Geometry check sheet. Reference: the model listing, model coordinates, mm. Face numbers are marked on the shaded views. Round coordinates to 2 decimals unless told otherwise and drop trailing zeros. Loops run counter-clockwise (first coordinate to the right, second up) from the corner with the lowest first, then second, coordinate; pieces in that order, holes last. Notation, with made-up numbers: M 28,35.5 L 64,35.5 A6 ccw 64,39.5 Z; hole C -14.5,46.25 d1. An arc over 180 degrees is marked long. Use one line per item in the form item = value. Start each with the question number.
1. Material ranges on line 1 (Y direction, x = 0, z = 5); line 2 (Z direction, x = 0, y = -42); line 3 (X direction, y = -3, z = 4.75), recorded low to high.
2. Draft check along Y on the marked faces 1, 2 and 3. Enter one of: pulls with the +Y half, pulls with the -Y half, needs draft (parallel to the pull), parting line crosses it, or undercut.
3. Cross-section at A-A (y = 0). Record the boundary of the cut face in (x, z).
4. Cross-section at C-C (y = -16). Record the boundary of the cut face in (x, z), then the cut area to 3 significant figures.
5. Go/stop test with flat-tipped pins: pin 1 (0.9 mm diameter, centred on y = 0.5, z = 4.5, fed in from -X); pin 2 (1.5 mm diameter, centred on x = 0, z = 4, fed in from +Y); pin 3 (1.5 mm diameter, centred on y = 22, z = 6, fed in from +X). Record where each tip stops, or that it passes through.
6. Cross-section at B-B (z = 4). Record the boundary of the cut face in (x, y), then the cut area to 3 significant figures.
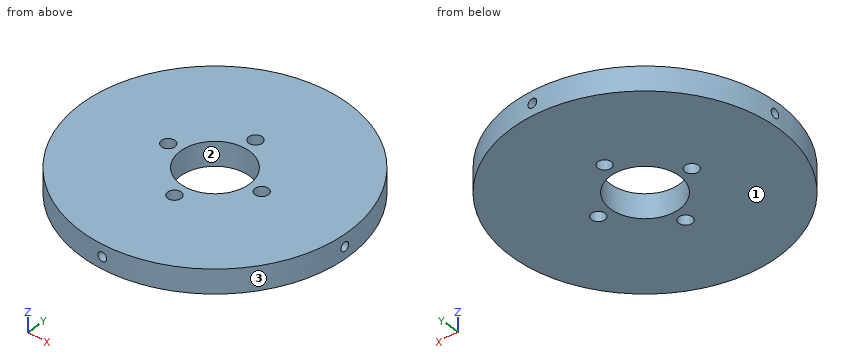
Autodesk Inventor part; units mm, degrees
ref_plane "作業平面1" through (45, 0, 0) normal (1, 0, 0) x (0, 1, 0)
ref_plane "作業平面2" through (-45, 0, 0) normal (1, 0, 0) x (0, 1, 0)
ref_plane "作業平面3" through (0, 45, 0) normal (0, 1, 0) x (-1, 0, 0)
sketch "スケッチ1" plane through (0, 0, 0) normal (0, 0, 1) x (1, 0, 0)
  circle A0 centre (0, 0) radius 44.5
  circle A1 centre (0, 0) radius 11.5
  dimension "d0" = 89
  dimension "d1" = 23
extrude "押し出し1" add sketch "スケッチ1" along normal blind 8
sketch "スケッチ2" plane through (0, 0, 8) normal (0, 0, 1) x (1, 0, 0)
  line L0 (0, 0) -> (0, 16) construction
  circle A0 centre (0, 16) radius 2.25
  circle A1 centre (-16, 0) radius 2.25
  circle A2 centre (0, -16) radius 2.25
  circle A3 centre (16, 0) radius 2.25
  dimension "d4" = 16
  dimension "d5" = 4.5
  dimension "d8" = 360
extrude "押し出し2" cut sketch "スケッチ2" against normal blind 8
ref_plane "作業平面1" through (45, 0, 0) normal (1, 0, 0) x (0, 1, 0)
sketch "スケッチ3" plane through (45, 0, 0) normal (1, 0, 0) x (0, 1, 0)
  line L0 (0, 0) -> (0, 4) construction
  circle A0 centre (0, 4) radius 1.5
  dimension "d13" = 4
  dimension "d14" = 3
extrude "押し出し3" cut sketch "スケッチ3" against normal blind 5
ref_plane "作業平面2" through (-45, 0, 0) normal (1, 0, 0) x (0, 1, 0)
sketch "スケッチ4" plane through (-45, 0, 0) normal (1, 0, 0) x (0, 1, 0)
  line L0 (0, 0) -> (0, 4) construction
  circle A0 centre (0, 4) radius 1.5
  dimension "d20" = 4
  dimension "d21" = 3
extrude "押し出し4" cut sketch "スケッチ4" along normal blind 5
ref_plane "作業平面3" through (0, 45, 0) normal (0, 1, 0) x (-1, 0, 0)
sketch "スケッチ5" plane through (0, 45, 0) normal (0, 1, 0) x (-1, 0, 0)
  line L0 (0, 0) -> (0, 4) construction
  circle A0 centre (0, 4) radius 1.5
  dimension "d25" = 4
  dimension "d26" = 3
extrude "押し出し5" cut sketch "スケッチ5" against normal blind 5
ref_plane "作業平面4" through (0, -45, 0) normal (0, 1, 0) x (-1, 0, 0)
sketch "スケッチ6" plane through (0, -45, 0) normal (0, 1, 0) x (-1, 0, 0)
  line L0 (0, 0) -> (0, 4) construction
  circle A0 centre (0, 4) radius 1.5
  dimension "d30" = 4
  dimension "d31" = 3
extrude "押し出し6" cut sketch "スケッチ6" along normal blind 5
thread "ねじ2"
thread "ねじ3"
thread "ねじ4"
thread "ねじ5"
properties part number "Bottom1"
Reported:
q1.line_1 = -40 to -18.25, -13.75 to -11.5, 11.5 to 13.75, 18.25 to 40
q1.line_2 = 0 to 2.5, 5.5 to 8
q1.line_3 = -44.4 to -11.1, 11.1 to 44.4
q2.face_1 = needs draft
q2.face_2 = undercut
q2.face_3 = parting line crosses it
q3.outline = M -44.5,0 L -18.25,0 L -18.25,8 L -44.5,8 L -44.5,5.5 L -40,5.5 L -40,2.5 L -44.5,2.5 Z; M -13.75,0 L -11.5,0 L -11.5,8 L -13.75,8 Z; M 11.5,0 L 13.75,0 L 13.75,8 L 11.5,8 Z; M 18.25,0 L 44.5,0 L 44.5,2.5 L 40,2.5 L 40,5.5 L 44.5,5.5 L 44.5,8 L 18.25,8 Z
q4.outline = M -41.52,0 L -2.25,0 L -2.25,8 L -41.52,8 Z; M 2.25,0 L 41.52,0 L 41.52,8 L 2.25,8 Z
q4.area = 628 mm²
q5.pin_1 = -40
q5.pin_2 = 40
q5.pin_3 = 39.1
q6.outline = M -44.47,-1.5 A44.5 ccw -1.5,-44.47 L -1.5,-40 L 1.5,-40 L 1.5,-44.47 A44.5 ccw 44.47,-1.5 L 40,-1.5 L 40,1.5 L 44.47,1.5 A44.5 ccw 1.5,44.47 L 1.5,40 L -1.5,40 L -1.5,44.47 A44.5 ccw -44.47,1.5 L -40,1.5 L -40,-1.5 Z; hole C -16,0 d4.5; hole C 0,0 d23; hole C 0,-16 d4.5; hole C 0,16 d4.5; hole C 16,0 d4.5
q6.area = 5,690 mm²
